CAD build for the part. Positions are in the model's coordinates, mm. A direction names the side the tool comes from. Coordinates: 2 decimals unless noted, no trailing zeros. Order: outer loops, then holes, each group sorted by start corner. A loop starts at its lowest first (then second) coordinate and runs counter-clockwise, first axis right, second up. Notation, with made-up numbers: M -5,38.25 L -1,38.25 A20 ccw -1,65.25 Z; hole C -27.5,79 d9. An arc over 180 degrees is marked long. One line per item, written item: value.
from build123d import *

# Parameters (mm, degrees)
F0_W         = 30
F0_H         = 30
F1_DEPTH     = 4
F2_W         = 3
F2_H         = 10
F3_DEPTH     = 15
F5_DEPTH     = 15
F6_W         = 5
F6_H         = 3
F7_DEPTH     = 3
F8_R         = 2.99999
F9_R         = 1.65
F10_DEPTH    = 25
F11_W        = 3
F11_H        = 3
F12_DEPTH    = 12.5
F13_R        = 2.99999
F14_R        = 2.5
F15_DEPTH    = 18.8
F16_T1_DEPTH = 39.6571957465
F16_T3_DEPTH = 39.6571957465


# Not quite as in the source:
# - a fillet or chamfer that OpenCascade refuses, or shapes differently, is made with other operations: its cross-section is extruded or revolved along the edge and cut away or added
# - a fillet or chamfer is up to 0.001 mm smaller than in the source, because OpenCascade refuses the exact size


with BuildPart() as f1:
    # F0 (on Top) → F1 (new body)
    with BuildSketch(Plane.XY):
        Rectangle(F0_W, F0_H)
    extrude(amount=-F1_DEPTH)

    # F2 (on Front) → F3 (join, symmetric)
    with BuildSketch(Plane.XZ):
        with Locations((-13.5, 5)):
            Rectangle(F2_W, F2_H)
        with Locations((13.5, 5)):
            Rectangle(F2_W, F2_H)
    extrude(amount=F3_DEPTH, both=True)

    # F4 (on Front) → F5 (join, symmetric)
    with BuildSketch(Plane.XZ):
        with BuildLine():
            Line((-12, 6.7849478247), (-12, 9))
            ThreePointArc((-12, 9), (-12.0709686948, 7.8924739124), (-12, 6.7849478247))
        make_face()
        with BuildLine():
            ThreePointArc((-7, 0), (-10.3790782907, 2.7446588419), (-12, 6.7849478247))
            Line((-12, 6.7849478247), (-12, 0))
            Line((-12, 0), (-7, 0))
        make_face()
        with BuildLine():
            Line((12, 0), (12, 6.7849478247))
            ThreePointArc((12, 6.7849478247), (10.3790782907, 2.7446588419), (7, 0))
            Line((7, 0), (12, 0))
        make_face()
        with BuildLine():
            ThreePointArc((12, 6.7849478247), (12.0709686948, 7.8924739124), (12, 9))
            Line((12, 9), (12, 6.7849478247))
        make_face()
    extrude(amount=F5_DEPTH, both=True)

    # F6 (on Front) → F7 (join, symmetric)
    with BuildSketch(Plane.XZ):
        with Locations((-17.5, -2.5)):
            Rectangle(F6_W, F6_H)
        with Locations((17.5, -2.5)):
            Rectangle(F6_W, F6_H)
    extrude(amount=F7_DEPTH, both=True)

    # F8 (radius 3 in the source; OpenCascade refuses exactly that, so slightly less here)
    f8_edges = [f1.edges().sort_by_distance(p)[0] for p in [
        (-20, 3, -2.5),
        (-20, -3, -2.5),
        (20, 3, -2.5),
        (20, -3, -2.5),
    ]]
    fillet(f8_edges, radius=F8_R)

    # F9 (on Top) → F10 (cut)
    with BuildSketch(Plane.XY):
        with Locations((-17.5, 0)):
            Circle(F9_R)
        with Locations((17.5, 0)):
            Circle(F9_R)
    extrude(amount=-F10_DEPTH, mode=Mode.SUBTRACT)

    # F11 (on Front) → F12 (join, symmetric)
    with BuildSketch(Plane.XZ):
        with Locations((-13.5, 11.5)):
            Rectangle(F11_W, F11_H)
        with Locations((13.5, 11.5)):
            Rectangle(F11_W, F11_H)
    extrude(amount=F12_DEPTH, both=True)

    # F13 (radius 3 in the source; OpenCascade refuses exactly that, so slightly less here)
    f13_edges = [f1.edges().sort_by_distance(p)[0] for p in [
        (-13.5, -12.5, 13),
        (-13.5, 12.5, 13),
        (13.5, -12.5, 13),
        (13.5, 12.5, 13),
    ]]
    fillet(f13_edges, radius=F13_R)

    # F14 (on Right) → F15 (cut, symmetric)
    with BuildSketch(Plane.YZ):
        with Locations((7, 9.75)):
            Circle(F14_R)
    extrude(amount=F15_DEPTH, both=True, mode=Mode.SUBTRACT)

    # F16: fillet of radius 12 on 4 edges, made by hand

    # F16_s2 → F16_t1 (cut)
    with BuildSketch(Plane.YZ.offset(-6.3285978733)):
        with BuildLine():
            ThreePointArc((15, 2.6685608507), (14.3578166916, 6.5415441969), (12.5, 10))
            Line((12.5, 10), (15, 10))
            Line((15, 10), (15, 2.6685608507))
        make_face()
        with BuildLine():
            ThreePointArc((-15, 2.6685608507), (-14.3578166916, 6.5415441969), (-12.5, 10))
            Line((-12.5, 10), (-15, 10))
            Line((-15, 10), (-15, 2.6685608507))
        make_face()
    extrude(amount=F16_T1_DEPTH, mode=Mode.SUBTRACT)

    # F16_s4 → F16_t3 (cut)
    with BuildSketch(Plane.YZ.offset(-33.3285978733)):
        with BuildLine():
            ThreePointArc((-12.5, 10), (-14.3578166916, 6.5415441969), (-15, 2.6685608507))
            Line((-15, 2.6685608507), (-15, 10))
            Line((-15, 10), (-12.5, 10))
        make_face()
        with BuildLine():
            ThreePointArc((12.5, 10), (14.3578166916, 6.5415441969), (15, 2.6685608507))
            Line((15, 2.6685608507), (15, 10))
            Line((15, 10), (12.5, 10))
        make_face()
    extrude(amount=F16_T3_DEPTH, mode=Mode.SUBTRACT)


solid = f1.part
Q1. Slice it at D-D (z = 2). List the corners of the cut face in (x, y).
Recorded:
outline: M -15,-15 L -9.76,-15 L -9.76,15 L -15,15 Z; M 9.76,-15 L 15,-15 L 15,15 L 9.76,15 Z
Q2. Slice it at C-C (x = 17.5). List the corners of the cut face in (y, z).
Recorded:
outline: M -2.96,-4 L -1.65,-4 L -1.65,-1 L -2.96,-1 Z; M 1.65,-4 L 2.96,-4 L 2.96,-1 L 1.65,-1 Z
Q3. Slice it at B-B (z = -1.75). Give the number of separate pieces and of enclosed holes in the cut face, plus the area to 3 significant figures.
Recorded:
separate pieces: 1
enclosed holes: 2
area: 935 mm^2
Q4. Slice it at A-A (y = 7). List the corners of the cut face in (x, z), plus the area to 3 significant figures.
Recorded:
outline: M -15,-4 L 15,-4 L 15,7.25 L 12,7.25 L 12,6.78 A8.68 cw 7,0 L -7,0 A8.68 cw -12,6.78 L -12,7.25 L -15,7.25 Z; M -15,12.25 L -12,12.25 L -12,13 L -15,13 Z; M 12,12.25 L 15,12.25 L 15,13 L 12,13 Z
area: 189 mm^2
Q5. Mould opens along X. For faces 1 (the face through (13.52, 8.15, 7.53)), 2 (the face through (19.074, 0.496, -2.479)), 3 (the face through (-19.1, 2.14, -2.48)) say: released by +X, released by -X, zero draft, split by the parting line, or undercut.
Recorded:
face 1: zero draft
face 2: undercut
face 3: released by -X
Q6. Drill centre lines: line 1 along X through (y, z) = (-9, 11.25); line 2 along Z through (x, y) = (-13, 7); line 3 along Y through (x, z) = (-17, -2.75). Where is each one in solid material? Low to high.
Recorded:
line 1: x = -15 to -12, 12 to 15
line 2: z = -4 to 7.25, 12.25 to 13
line 3: y = -3 to -1.57, 1.57 to 3
Q7. Pin check, flat tips, straight feed: pin 1 Ø1.6 at (x, z) = (16.5, -2.5) entering from -Y; pin 2 Ø1 at (x, z) = (16, -2.5) entering from +Y; pin 3 Ø7 at (y, z) = (-3.5, 9) entering from -X; pin 4 Ø4 at (y, z) = (7, 9.75) entering from -X. Stop position of each tip, or through.
Recorded:
pin 1: stops at y = -3
pin 2: stops at y = 3
pin 3: stops at x = -15
pin 4: passes through
Q8. Which spindle directions (+Z, -Z, +X, -X, +Y, -Y) get a long thin tool onto all of the face, cutting with end or side? Do faces 4 (the face through (-16, -3, -2)), 5 (the face through (16, 3, -2)), 6 (the face through (16, 1, -1)), 7 (the face through (0, 0, 0)). Say none if no direction does.
Recorded:
face 4: +Z, -Z, -X, -Y
face 5: +Z, -Z, +X, +Y
face 6: +Z, +X, +Y, -Y
face 7: +Z, +Y, -Y
